Here's how the part is built. I have some questions about the finished solid (model axes, mm). A direction names the side the tool comes from. Coordinates: 2 decimals unless noted, no trailing zeros. Write each loop counter-clockwise with the first axis right and the second up, starting at its lowest first coordinate (ties: lowest second). Pieces come first, ordered by that corner, then holes. Notation, with made-up numbers: M 88.25,13.5 L 117.25,13.5 A12 ccw 117.25,31.5 Z; hole C -10.5,-2.5 d9. An arc over 180 degrees is marked long. Use a Markdown table: item, result.
```python
from build123d import *

# Parameters (mm, degrees)
SKETCH1_R           = 1.6
BOSS_EXTRUDE1_DEPTH = 2


with BuildPart() as part:
    # Sketch1 → Boss-Extrude1 (new body)
    with BuildSketch(Plane.XY):
        Polygon((-39.5636369, 18.881491211), (55.4363631, 18.881491211), (55.4363631, -41.118508789), (-39.5636369, -41.118508789), (-39.5636369, -31.118508789), (-27.5636369, -31.118508789), (-27.5636369, -12.118508789), (-39.5636369, -12.118508789), (-39.5636369, -10.118508789), (-27.5636369, -10.118508789), (-27.5636369, 8.881491211), (-39.5636369, 8.881491211), align=None)
        with Locations((20.4363631, 13.881491211)):
            Circle(SKETCH1_R, mode=Mode.SUBTRACT)
        with Locations((20.4363631, -36.118508789)):
            Circle(SKETCH1_R, mode=Mode.SUBTRACT)
        with Locations((-36.5636369, 15.881491211)):
            Circle(SKETCH1_R, mode=Mode.SUBTRACT)
        with Locations((52.4363631, 15.881491211)):
            Circle(SKETCH1_R, mode=Mode.SUBTRACT)
        with Locations((-36.5636369, -38.118508789)):
            Circle(SKETCH1_R, mode=Mode.SUBTRACT)
        with Locations((52.4363631, -38.118508789)):
            Circle(SKETCH1_R, mode=Mode.SUBTRACT)
        with BuildLine():
            Line((7.9363631, -4.118508789), (32.9363631, -4.118508789))
            ThreePointArc((32.9363631, -4.118508789), (34.350576663, -4.704295227), (34.9363631, -6.118508789))
            Line((34.9363631, -6.118508789), (34.9363631, -16.118508789))
            ThreePointArc((34.9363631, -16.118508789), (34.350576663, -17.532722351), (32.9363631, -18.118508789))
            Line((32.9363631, -18.118508789), (7.9363631, -18.118508789))
            ThreePointArc((7.9363631, -18.118508789), (6.522149538, -17.532722351), (5.9363631, -16.118508789))
            Line((5.9363631, -16.118508789), (5.9363631, -6.118508789))
            ThreePointArc((5.9363631, -6.118508789), (6.522149538, -4.704295227), (7.9363631, -4.118508789))
        make_face(mode=Mode.SUBTRACT)
    extrude(amount=BOSS_EXTRUDE1_DEPTH)


solid = part.part
```
1. Suppose I cut it at A-A on x = -31. Write out the boundary of the cut face in (y, z).
Answers follow:
| item | result |
|---|---|
| outline | M -41.12,0 L -31.12,0 L -31.12,2 L -41.12,2 Z; M -12.12,0 L -10.12,0 L -10.12,2 L -12.12,2 Z; M 8.88,0 L 18.88,0 L 18.88,2 L 8.88,2 Z |
2. Suppose I cut it at B-B on y = -13.5. Write out the boundary of the cut face in (x, z), and give its area (3 significant figures).
Answers follow:
| item | result |
|---|---|
| outline | M -27.56,0 L 5.94,0 L 5.94,2 L -27.56,2 Z; M 34.94,0 L 55.44,0 L 55.44,2 L 34.94,2 Z |
| area | 108 mm2 |
3. Suppose I cut it at D-D on z = 0.95. Write out the boundary of the cut face in (x, y).
Answers follow:
| item | result |
|---|---|
| outline | M -39.56,-41.12 L 55.44,-41.12 L 55.44,18.88 L -39.56,18.88 L -39.56,8.88 L -27.56,8.88 L -27.56,-10.12 L -39.56,-10.12 L -39.56,-12.12 L -27.56,-12.12 L -27.56,-31.12 L -39.56,-31.12 Z; hole C -36.56,-38.12 d3.2; hole C -36.56,15.88 d3.2; hole M 5.94,-16.12 A2 ccw 7.94,-18.12 L 32.94,-18.12 A2 ccw 34.94,-16.12 L 34.94,-6.12 A2 ccw 32.94,-4.12 L 7.94,-4.12 A2 ccw 5.94,-6.12 Z; hole C 20.44,-36.12 d3.2; hole C 20.44,13.88 d3.2; hole C 52.44,-38.12 d3.2; hole C 52.44,15.88 d3.2 |
4. We'd pull the mould along X, two halves only. Please class faces 4 (the face through (-2, -11, 0)), 5 (the face through (-27.564, -22, 1)), 6 (the face through (52.09, 14.32, 0.99)): +X half, -X half, draft (parallel to the pull), parting line (faces both ways), or undercut.
Answers follow:
| item | result |
|---|---|
| face 4 | draft |
| face 5 | -X half |
| face 6 | undercut |
5. Which directions (+Z, -Z, +X, -X, +Y, -Y) give clear straight access to the entire face, cutting with the end or side of a thin tool? Please do faces 1 (the face through (-39.564, -11, 1)), 2 (the face through (34.936, -11, 1)), 3 (the face through (-34, -10.119, 1)).
Answers follow:
| item | result |
|---|---|
| face 1 | +Z, -Z, -X, +Y, -Y |
| face 2 | +Z, -Z |
| face 3 | +Z, -Z, -X |
6. I need wall thicknesses on probe 1 along X at (y, z) = (16, 1); probe 2 along Y at (x, z) = (-28.5, 1.4); probe 3 along Y at (x, z) = (18, 1.55). Which ranges of each line are inside material? Lowest first, please.
Answers follow:
| item | result |
|---|---|
| probe 1 | x = -39.56 to -38.16, -34.97 to 50.84, 54.03 to 55.44 |
| probe 2 | y = -41.12 to -31.12, -12.12 to -10.12, 8.88 to 18.88 |
| probe 3 | y = -41.12 to -18.12, -4.12 to 18.88 |
7. Suppose I cut it at C-C on x = 15. Write out the boundary of the cut face in (y, z).
Answers follow:
| item | result |
|---|---|
| outline | M -41.12,0 L -18.12,0 L -18.12,2 L -41.12,2 Z; M -4.12,0 L 18.88,0 L 18.88,2 L -4.12,2 Z |
